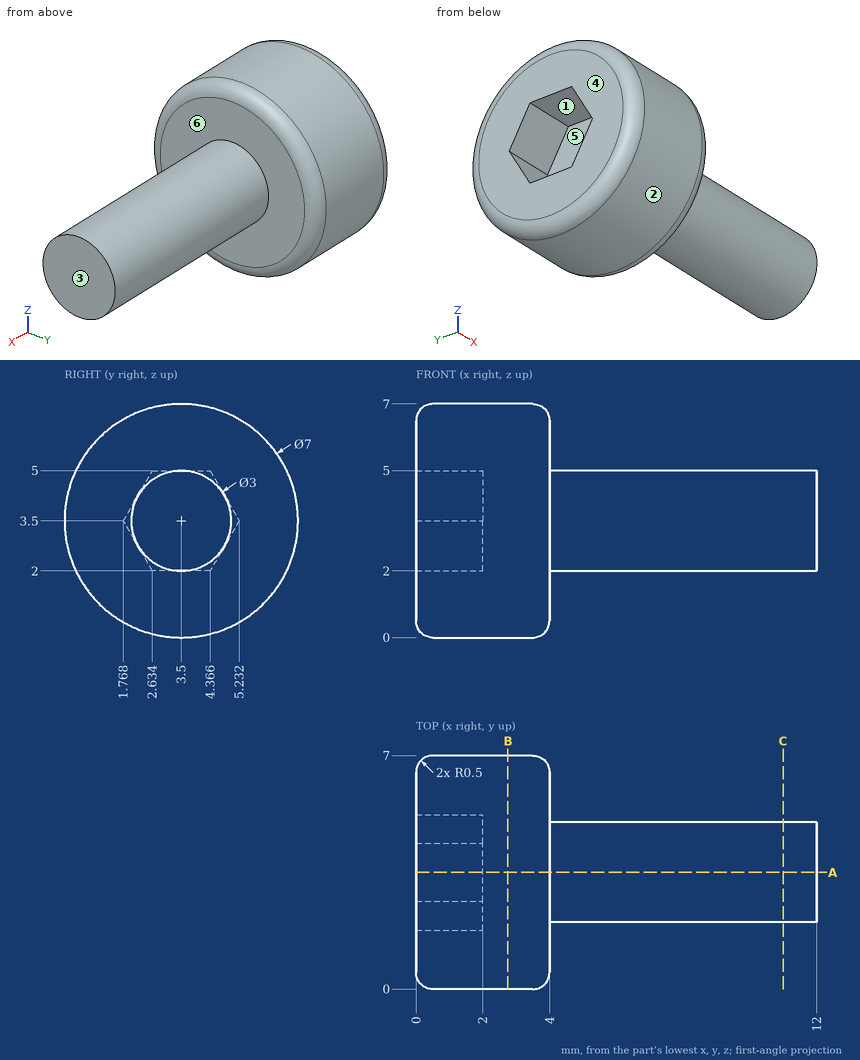
Print and shaded views of the part. All mm, measured from the part's lowest x, y and z. A direction names the side the tool comes from. Give positions to 0.01 mm unless a question says otherwise; leave off trailing zeros. Write each loop counter-clockwise with the first axis right and the second up, starting at its lowest first coordinate (ties: lowest second). Pieces come first, ordered by that corner, then holes. Notation, with made-up numbers: M 82,21.25 L 132,21.25 A21 cw 132,39.25 Z; hole C 44,-27.5 d9. An arc over 180 degrees is marked long. Use a Markdown table: item, result.
1) Cut at A-A (y = 3.5). List the corners of the cut face in (x, z), and give its area (3 significant figures).
Responses:
| item | result |
|---|---|
| outline | M 0,0.5 A0.5 ccw 0.5,0 L 3.5,0 A0.5 ccw 4,0.5 L 4,2 L 12,2 L 12,5 L 4,5 L 4,6.5 A0.5 ccw 3.5,7 L 0.5,7 A0.5 ccw 0,6.5 L 0,5 L 2,5 L 2,2 L 0,2 Z |
| area | 45.8 mm2 |
2) Pin check, flat tips, straight feed: pin 1 (1.5 mm diameter, centred on y = 3, z = 4, fed in from -X); pin 2 (1.5 mm diameter, centred on x = 8.5, z = 4.5, fed in from -Y); pin 3 (1 mm diameter, centred on x = 1.5, z = 6, fed in from +Y). Stop position of each tip, or through.
Responses:
| item | result |
|---|---|
| pin 1 | stops at x = 2 |
| pin 2 | stops at y = 2.02 |
| pin 3 | stops at y = 6.37 |
3) Tool access for the marked faces 4, 5 and 6: list every direction of +Z, -Z, +X, -X, +Y, -Y with a clear straight run to the whole face (end or side of a thin tool).
Responses:
| item | result |
|---|---|
| face 4 | +Z, -Z, -X, +Y, -Y |
| face 5 | -X |
| face 6 | +X |
4) Pull direction Z, two halves, no side cores. Call the marked faces 1, 2 and 3: +Z half, -Z half, draft (parallel to the pull), parting line (faces both ways), or undercut.
Responses:
| item | result |
|---|---|
| face 1 | undercut |
| face 2 | parting line |
| face 3 | draft |
5) Cut at C-C (x = 11). List the corners of the cut face in (y, z), and give its area (3 significant figures).
Responses:
| item | result |
|---|---|
| outline | C 3.5,3.5 d3 |
| area | 7.07 mm2 |
6) Drill centre lines: line 1 (X direction, y = 5, z = 2.5); line 2 (X direction, y = 3, z = 2.25); line 3 (Y direction, x = 7.5, z = 3.5). Where is each one in solid material? Low to high. Write a range as from..to.
Responses:
| item | result |
|---|---|
| line 1 | x = 0..4 |
| line 2 | x = 2..12 |
| line 3 | y = 2..5 |
7) Cut at B-B (x = 2.75). List the corners of the cut face in (y, z).
Responses:
| item | result |
|---|---|
| outline | C 3.5,3.5 d7 |
